Geometry: final body of the model. Coordinates: model frame, mm. Face numbers are marked on the shaded views. A direction names the side the tool comes from. Round coordinates to 2 decimals unless told otherwise and drop trailing zeros. Write each loop counter-clockwise with the first axis right and the second up, starting at its lowest first coordinate (ties: lowest second). Pieces come first, ordered by that corner, then holes. Notation, with made-up numbers: (72.5, -11) - (79.5, -11) arc R27 ccw to (79.5, 7) - close; hole circle Ø10 at (1.25, 83.5). An arc over 180 degrees is marked (long way). Write each question's results on one line, items separated by ' | '.
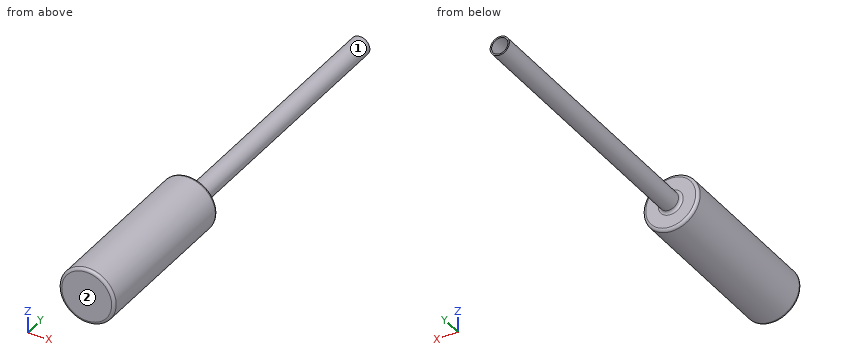
from build123d import *

# Parameters (mm, degrees)
F2_T = -2.54
F3_R = 5.08


with BuildPart() as f1:
    # F0 (on Right) → F1 (revolve)
    with BuildSketch(Plane.YZ):
        Polygon((78.3833178774, 68.3245788985), (-221.6166821226, 68.3245788985), (-221.6166821226, 18.3245788985), (578.3833178774, 18.3245788985), (578.3833178774, 35.5585788985), (78.3833178774, 35.5585788985), align=None)
    revolve(axis=Axis((0, 178.3833178774, 18.3245788985), (0, 1, 0)))

    # F2
    f2_openings = [f1.faces().sort_by_distance(p)[0] for p in [
        (0, 578.383318, 18.324579),
    ]]
    offset(amount=F2_T, openings=f2_openings, kind=Kind.INTERSECTION)

    # F3
    f3_edges = [f1.edges().sort_by_distance(p)[0] for p in [
        (0, 78.383318, -31.675421),
        (0, 78.383318, 1.090579),
        (0, -221.616682, -31.675421),
    ]]
    fillet(f3_edges, radius=F3_R)


solid = f1.part
Q1. Ray query, line 1 along Y through (x, z) = (-15.5, 55); line 2 along Y through (x, z) = (45.5, 37.5); line 3 along X through (y, z) = (-140.5, 21). Return the intervals inside material, ascending.
Answer block:
line 1: -221.62 to -219.08, 75.84 to 78.38 | line 2: -218.98 to 75.74 | line 3: -49.93 to -47.38, 47.38 to 49.93
Q2. Access query for the marked faces 1 and 2. Directions: +Z, -Z, +X, -X, +Y, -Y. A direction counts if a zero-diameter tool reaches every point of the face in a straight line with its end or side. Return the directions, or none.
Answer block:
face 1: +Y | face 2: +Z, -Z, +X, -X, -Y
Q3. Section query C-C, the plane y = -141.5. Return loops of the section in (x, z).
Answer block:
outline: circle Ø100 at (0, 18.32); hole circle Ø94.92 at (0, 18.32)
Q4. Section query B-B, the plane x = 0. Return loops of the section in (y, z).
Answer block:
outline: (-221.62, -26.6) arc R5.08 ccw to (-216.54, -31.68) - (73.3, -31.68) arc R5.08 ccw to (78.38, -26.6) - (78.38, -3.99) arc R5.08 cw to (83.46, 1.09) - (578.38, 1.09) - (578.38, 3.63) - (75.84, 3.63) - (75.84, -29.14) - (-219.08, -29.14) - (-219.08, 65.78) - (75.84, 65.78) - (75.84, 33.02) - (578.38, 33.02) - (578.38, 35.56) - (83.46, 35.56) arc R5.08 cw to (78.38, 40.64) - (78.38, 63.24) arc R5.08 ccw to (73.3, 68.32) - (-216.54, 68.32) arc R5.08 ccw to (-221.62, 63.24) - close
Q5. Pin query (flat end, axial travel): pin 1 (10 mm diameter, centred on y = 42, z = 25, fed in from +X); pin 2 (4 mm diameter, centred on x = 6.5, y = 129.5, fed in from +Z); pin 3 (10 mm diameter, centred on y = 122, z = -1, fed in from -X). Return the tip coordinate at first contact, or that it passes through.
Answer block:
pin 1: x = 49.97 | pin 2: z = 34.96 | pin 3: x = -9.58
Q6. Section query A-A, the plane y = 374. Return loops of the section in (x, z).
Answer block:
outline: circle Ø34.47 at (0, 18.32); hole circle Ø29.39 at (0, 18.32)
